Source: CAD feature listing. Evaluate the final solid. Frame: model axes, mm. Give positions to 0.01 mm unless a question says otherwise; leave off trailing zeros. Order: outer loops, then holes, each group sorted by start corner. A loop starts at its lowest first (then second) coordinate and runs counter-clockwise, first axis right, second up. Notation, with made-up numbers: M -6.5,88.25 L 15.5,88.25 A28 cw 15.5,112.25 Z; hole C 79.5,25 d5. An arc over 180 degrees is marked long. Answer as a JSON object with one key per item and string values. Group by question number.
1. Pin query (flat end, axial travel): P1, Ø2.5, axis at x = -26.31, z = 9.58, coming from the +Y side; P2, Ø2, axis at x = 7, y = 2, coming from the -Z side; P3, Ø2, axis at x = -14, y = 3, coming from the +Z side. Return the tip coordinate at first contact, or that it passes through.
2. Material intervals for L1, parallel to Z at x = 0, y = 2.7; L2, parallel to X at y = 2, z = 22.5; L3, parallel to X at y = 1.5, z = -10.5, sorted ascending. Write a range as [from, to].
3. Pull-direction query (X, two-part tool) for faces 1 (the cylindrical face through (-24.065, 1.972, 26.071)), 2 (the flat face through (10, 4, -18)); classes: +X half, -X half, draft (parallel to the pull), parting line (faces both ways), or undercut.
4. Section query D-D (x = 37). Output: boundary loops of the cut face in (y, z), plus the area to 3 significant figures.
5. Section query C-C (z = -13.5). Output: boundary loops of the cut face in (x, y).
6. Section query B-B (y = 1.15). Count the separate pieces of the cut face and the enclosed holes in it, plus the area to 3 significant figures.
7. Section query A-A (x = 0). Output: boundary loops of the cut face in (y, z), plus the area to 3 significant figures.
Autodesk Inventor part; units mm, degrees
ref_plane "YZ Plane" through (0, 0, 0) normal (1, 0, 0) x (0, 1, 0)
ref_plane "XZ Plane" through (0, 0, 0) normal (0, 1, 0) x (-1, 0, 0)
ref_plane "XY Plane" through (0, 0, 0) normal (0, 0, 1) x (1, 0, 0)
sketch "Sketch1" plane through (0, 0, 0) normal (0, 1, 0) x (-1, 0, 0)
  circle A0 centre (0, 0) radius 42
  circle A1 centre (0, 0) radius 19.5
  circle A2 centre (0, -37) radius 2.1
  circle A3 centre (26.163, -26.163) radius 2.1
  circle A4 centre (37, 0) radius 2.1
  circle A5 centre (26.163, 26.163) radius 2.1
  circle A6 centre (0, 37) radius 2.1
  circle A7 centre (-26.163, 26.163) radius 2.1
  circle A8 centre (-37, 0) radius 2.1
  circle A9 centre (-26.163, -26.163) radius 2.1
  circle A10 centre (-4.8621, -27.5746) radius 2.1
  circle A11 centre (4.8621, -27.5746) radius 2.1
  circle A12 centre (14, -24.2487) radius 2.1
  circle A13 centre (21.4492, -17.9981) radius 2.1
  circle A14 centre (26.3114, -9.5766) radius 2.1
  circle A15 centre (28, 0) radius 2.1
  circle A16 centre (26.3114, 9.5766) radius 2.1
  circle A17 centre (21.4492, 17.9981) radius 2.1
  circle A18 centre (14, 24.2487) radius 2.1
  circle A19 centre (4.8621, 27.5746) radius 2.1
  circle A20 centre (-4.8621, 27.5746) radius 2.1
  circle A21 centre (-14, 24.2487) radius 2.1
  circle A22 centre (-21.4492, 17.9981) radius 2.1
  circle A23 centre (-26.3114, 9.5766) radius 2.1
  circle A24 centre (-28, 0) radius 2.1
  circle A25 centre (-26.3114, -9.5766) radius 2.1
  circle A26 centre (-21.4492, -17.9981) radius 2.1
  circle A27 centre (-14, -24.2487) radius 2.1
  line L0 (0, 0) -> (-4.8621, -27.5746) construction
  line L1 (0, 0) -> (0, -11.0753) construction
  dimension "d2" = 84
  dimension "d3" = 39
  dimension "d4" = 4.2
  dimension "d5" = 37
  dimension "d6" = 360
  dimension "d9" = 4.2
  dimension "d10" = 28
  dimension "d11" = 360
  dimension "d12" = 10
extrude "Extrusion1" add sketch "Sketch1" along normal blind 4
properties part number "HousingExampleLid"
Answer sheet:
{
 "1": {"P1": "through", "P2": "z = -41.57", "P3": "z = 39.94"},
 "2": {"L1": "[-42, -39.1], [-34.9, -19.5], [19.5, 34.9], [39.1, 42]", "L2": "[-35.46, -15.16], [-12.84, 12.84], [15.16, 35.46]", "L3": "[-40.67, -28.2], [-24.43, -16.43], [16.43, 24.43], [28.2, 40.67]"},
 "3": {"face 1": "undercut", "face 2": "draft"},
 "4": {"outline": "M 0,-19.87 L 4,-19.87 L 4,-2.1 L 0,-2.1 Z; M 0,2.1 L 4,2.1 L 4,19.87 L 0,19.87 Z", "area": "142 mm^2"},
 "5": {"outline": "M -39.77,0 L -14.07,0 L -14.07,4 L -39.77,4 Z; M 14.07,0 L 39.77,0 L 39.77,4 L 14.07,4 Z"},
 "6": {"separate pieces": "1", "enclosed holes": "27", "area": "3,990 mm^2"},
 "7": {"outline": "M 0,-42 L 4,-42 L 4,-39.1 L 0,-39.1 Z; M 0,-34.9 L 4,-34.9 L 4,-19.5 L 0,-19.5 Z; M 0,19.5 L 4,19.5 L 4,34.9 L 0,34.9 Z; M 0,39.1 L 4,39.1 L 4,42 L 0,42 Z", "area": "146 mm^2"}
}
